The listing builds one solid part. Answer for the finished solid, in the listing's coordinates (mm). Round coordinates to 2 decimals unless told otherwise and drop trailing zeros. Order: outer loops, then holes, each group sorted by start corner. A loop starts at its lowest first (then second) coordinate and runs counter-clockwise, first axis right, second up. Notation, with made-up numbers: (50.25, 73.5) - (79.25, 73.5) arc R4 ccw to (79.25, 79.5) - close; hole circle Ø4 at (-40, 22.5). An arc over 180 degrees is marked (long way). Write item = value, one per line.
from build123d import *

# Parameters (mm, degrees)
BOX058_W          = 2
BOX058_H          = 12
BOX058_DEPTH      = 10
BOX059_W          = 2
BOX059_H          = 12
BOX059_DEPTH      = 10
CYLINDER061_R     = 6
CYLINDER061_DEPTH = 10


with BuildPart() as cube057:
    # Box058 → Box058 (new body)
    with BuildSketch(Plane(origin=(145.25, 105.25, -5), x_dir=(1, 0, 0), z_dir=(0, 0, 1))):
        with Locations((1, 6)):
            Rectangle(BOX058_W, BOX058_H)
    extrude(amount=BOX058_DEPTH)


with BuildPart() as cube058:
    # Box059 → Box059 (new body)
    with BuildSketch(Plane(origin=(132.5, 105.25, -5), x_dir=(1, 0, 0), z_dir=(0, 0, 1))):
        with Locations((1, 6)):
            Rectangle(BOX059_W, BOX059_H)
    extrude(amount=BOX059_DEPTH)


with BuildPart() as keyhole:
    # Cylinder061 → Cylinder061 (new body)
    with BuildSketch(Plane(origin=(139.86, 111.25, -5), x_dir=(1, 0, 0), z_dir=(0, 0, 1))):
        Circle(CYLINDER061_R)
    extrude(amount=CYLINDER061_DEPTH)

    # Cut072: cut Cube058
    add(cube058.part, mode=Mode.SUBTRACT)

    # Cut073: cut Cube057
    add(cube057.part, mode=Mode.SUBTRACT)


solid = keyhole.part
Q1. A flat-ended cylindrical pin translates along its axis: P1, Ø1.5, axis at x = 136, z = -0.5, coming from the -Y side. Find the tip coordinate at first contact, or state that the pin passes through.
Model answer:
P1 = 106.12
Q2. Find the intervals of material crossed by line 1 (Y direction, x = 139.75, z = 1.5); line 2 (Y direction, x = 137, z = 3.75); line 3 (X direction, y = 115.75, z = 2), in increasing order. Write a range as from..to.
Model answer:
line_1 = 105.25..117.25
line_2 = 105.98..116.52
line_3 = 135.89..143.83
Q3. Section B-B on x = 143.25 is taken. Determine the outline of the cut face in (y, z).
Model answer:
outline = (106.3, -5) - (116.2, -5) - (116.2, 5) - (106.3, 5) - close
Q4. Section A-A on z = -0.75 is taken. Determine the outline of the cut face in (x, y).
Model answer:
outline = (134.5, 108.55) arc R6 ccw to (145.25, 108.61) - (145.25, 113.89) arc R6 ccw to (134.5, 113.95) - close
